```python
from build123d import *

# Parameters (mm, degrees)
SKETCH1_W           = 21
SKETCH1_H           = 21
BOSS_EXTRUDE1_DEPTH = 5
BOSS_EXTRUDE2_DEPTH = 16
SKETCH3_R           = 2.1
CUT_EXTRUDE1_DEPTH  = 3
SKETCH4_R           = 2.1
CUT_EXTRUDE2_DEPTH  = 3
SKETCH5_R           = 2.1
CUT_EXTRUDE3_DEPTH  = 3
CUT_EXTRUDE4_DEPTH  = 3
CUT_EXTRUDE5_DEPTH  = 3
CUT_EXTRUDE6_DEPTH  = 3
CHAMFER1_SIZE       = 2
FILLET1_R           = 2


with BuildPart() as part:
    # Sketch1 → Boss-Extrude1 (new body)
    with BuildSketch(Plane.XY):
        with Locations((10.5, 10.5)):
            Rectangle(SKETCH1_W, SKETCH1_H)
    extrude(amount=BOSS_EXTRUDE1_DEPTH)

    # Sketch2 → Boss-Extrude2 (add)
    with BuildSketch(Plane.XY.offset(5)):
        Polygon((0, 21), (21, 21), (21, 0), (16, 0), (16, 16), (0, 16), align=None)
    extrude(amount=BOSS_EXTRUDE2_DEPTH)

    # Sketch3 → Cut-Extrude1 (cut)
    with BuildSketch(Plane(origin=(0, 21, 0), x_dir=(1, 0, 0), z_dir=(0, 1, 0))):
        with Locations((6, -15)):
            Circle(SKETCH3_R)
    extrude(amount=-CUT_EXTRUDE1_DEPTH, mode=Mode.SUBTRACT)

    # Sketch4 → Cut-Extrude2 (cut)
    with BuildSketch(Plane(origin=(21, 0, 0), x_dir=(0, 0, -1), z_dir=(1, 0, 0))):
        with Locations((-15, 6)):
            Circle(SKETCH4_R)
    extrude(amount=-CUT_EXTRUDE2_DEPTH, mode=Mode.SUBTRACT)

    # Sketch5 → Cut-Extrude3 (cut)
    with BuildSketch(Plane(origin=(0, 0, 0), x_dir=(-1, 0, 0), z_dir=(0, 0, -1))):
        with Locations((-6, 6)):
            Circle(SKETCH5_R)
    extrude(amount=-CUT_EXTRUDE3_DEPTH, mode=Mode.SUBTRACT)

    # Sketch6 → Cut-Extrude4 (cut)
    with BuildSketch(Plane.ZY.offset(-16)):
        Polygon((18.5, 3.979274058), (18.5, 8.020725942), (15, 10.041451884), (11.5, 8.020725942), (11.5, 3.979274058), (15, 1.958548116), align=None)
    extrude(amount=-CUT_EXTRUDE4_DEPTH, mode=Mode.SUBTRACT)

    # Sketch7 → Cut-Extrude5 (cut)
    with BuildSketch(Plane.XY.offset(5)):
        Polygon((9.5, 3.979274058), (9.5, 8.020725942), (6, 10.041451884), (2.5, 8.020725942), (2.5, 3.979274058), (6, 1.958548116), align=None)
    extrude(amount=-CUT_EXTRUDE5_DEPTH, mode=Mode.SUBTRACT)

    # Sketch8 → Cut-Extrude6 (cut)
    with BuildSketch(Plane.XZ.offset(-16)):
        Polygon((8.020725942, 11.5), (10.041451884, 15), (8.020725942, 18.5), (3.979274058, 18.5), (1.958548116, 15), (3.979274058, 11.5), align=None)
    extrude(amount=-CUT_EXTRUDE6_DEPTH, mode=Mode.SUBTRACT)

    # Chamfer1
    chamfer1_edges = [part.edges().sort_by_distance(p)[0] for p in [
        (10.5, 21, 0),
        (21, 10.5, 0),
        (21, 21, 10.5),
    ]]
    chamfer(chamfer1_edges, length=CHAMFER1_SIZE)

    # Fillet1
    fillet1_edges = [part.edges().sort_by_distance(p)[0] for p in [
        (8, 16, 5),
        (16, 8, 5),
        (16, 16, 13),
    ]]
    fillet(fillet1_edges, radius=FILLET1_R)


solid = part.part
```
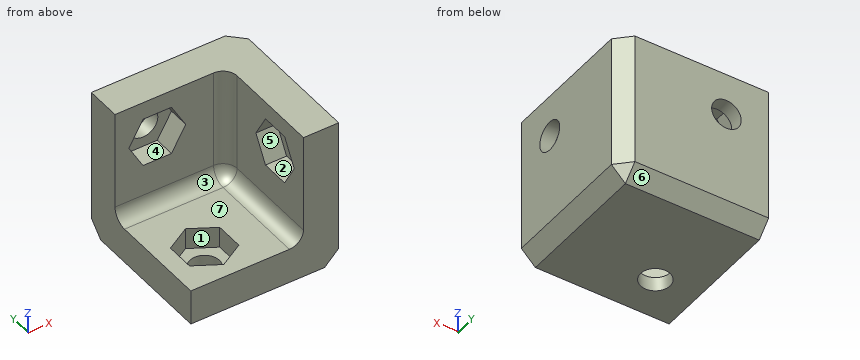
Source: CAD feature listing. Evaluate the final solid. Frame: model axes, mm. Face numbers are marked on the shaded views. A direction names the side the tool comes from. Round coordinates to 2 decimals unless told otherwise and drop trailing zeros. Order: outer loops, then holes, each group sorted by start corner. A loop starts at its lowest first (then second) coordinate and runs counter-clockwise, first axis right, second up. Notation, with made-up numbers: (63.5, -13) -> (107.5, -13) arc R13 cw to (107.5, 0) -> close; hole circle Ø5 at (21.5, 55.25). An arc over 180 degrees is marked (long way). Use CSV: the item, a comma, the result in double quotes.
(1) Section B-B on x = 16.75. Return the cut outline in (y, z), and give its area (3 significant figures).
Report:
outline,"(0, 0) -> (19, 0) -> (21, 2) -> (21, 21) -> (0, 21) -> close; hole (1.96, 15) -> (3.98, 11.5) -> (8.02, 11.5) -> (10.04, 15) -> (8.02, 18.5) -> (3.98, 18.5) -> close"
area,"397 mm^2"
(2) First-contact query: pin 1 Ø3.5 at (x, y) = (6.5, 6.5) entering from +Z; pin 2 Ø7.5 at (y, z) = (4.5, 15) entering from -X; pin 3 Ø4 at (x, y) = (6, 6) entering from +Z; pin 4 Ø6 at (x, z) = (5.5, 9.5) entering from -Y. Flat tips, straight axial feed; report the tip coordinate or a pass-through.
Report:
pin 1,"z = 2"
pin 2,"x = 16"
pin 3,"through"
pin 4,"y = 15.94"
(3) Pull-direction query (Y, two-part tool) for the marked faces 5, 6 and 7; classes: +Y half, -Y half, draft (parallel to the pull), parting line (faces both ways), or undercut.
Report:
face 5,"undercut"
face 6,"+Y half"
face 7,"draft"
(4) Section C-C on z = 8.5. Return the cut outline in (x, y), and give its area (3 significant figures).
Report:
outline,"(0, 16) -> (14, 16) arc R2 cw to (16, 14) -> (16, 0) -> (21, 0) -> (21, 19) -> (19, 21) -> (0, 21) -> close"
area,"184 mm^2"
(5) Ray query, L1, parallel to Z at x = 7.25, y = 18.25; L2, parallel to X at y = 3.5, z = 19; L3, parallel to Z at x = 6, y = 19.55. Return the intervals inside material, ascending.
Report:
L1,"0 to 11.5, 18.5 to 21"
L2,"16 to 21"
L3,"0.55 to 12.9, 17.1 to 21"
(6) Section A-A on y = 6. Return the cut outline in (x, z), and give its area (3 significant figures).
Report:
outline,"(0, 0) -> (3.9, 0) -> (3.9, 2) -> (2.5, 2) -> (2.5, 5) -> (0, 5) -> close; (8.1, 0) -> (19, 0) -> (21, 2) -> (21, 12.9) -> (19, 12.9) -> (19, 11.5) -> (16, 11.5) -> (16, 7) arc R2 cw to (14, 5) -> (9.5, 5) -> (9.5, 2) -> (8.1, 2) -> close; (16, 18.5) -> (19, 18.5) -> (19, 17.1) -> (21, 17.1) -> (21, 21) -> (16, 21) -> close"
area,"125 mm^2"
(7) Section D-D on x = 10.75. Return the cut outline in (y, z), and give its area (3 significant figures).
Report:
outline,"(0, 0) -> (19, 0) -> (21, 2) -> (21, 21) -> (16, 21) -> (16, 7) arc R2 cw to (14, 5) -> (0, 5) -> close"
area,"184 mm^2"
(8) Access query for the marked faces 1, 2, 3 and 4. Directions: +Z, -Z, +X, -X, +Y, -Y. A direction counts if a zero-diameter tool reaches every point of the face in a straight line with its end or side. Return the directions, or none.
Report:
face 1,"+Z"
face 2,"-X"
face 3,"+Z, -X, -Y"
face 4,"-Y"
